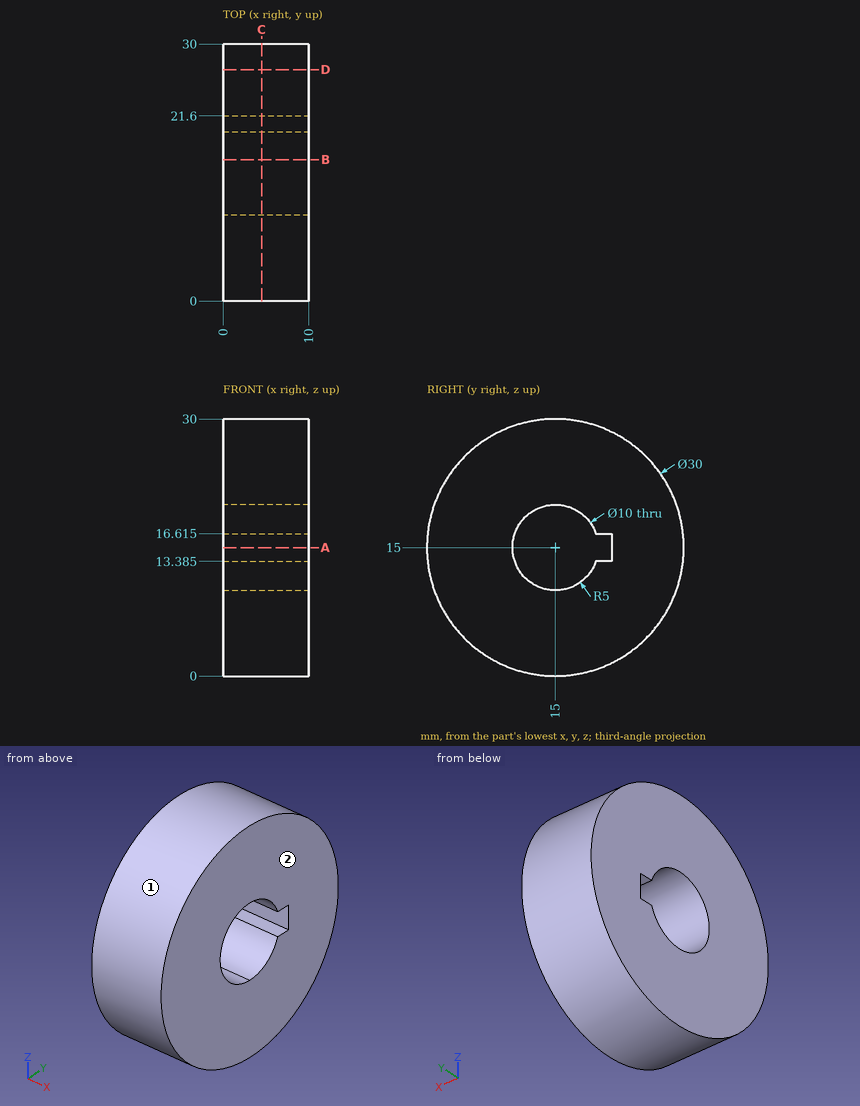
Geometry: see drawing. Coordinates: mm, zero at the bounding-box minimum. Round coordinates to 2 decimals unless told otherwise and drop trailing zeros. Loops run counter-clockwise (first coordinate to the right, second up) from the corner with the lowest first, then second, coordinate; pieces in that order, holes last. Notation, with made-up numbers: (52.5, -30.75) -> (111.5, -30.75) arc R38 cw to (111.5, 7.25) -> close; hole circle Ø5 at (19, 51). An arc over 180 degrees is marked (long way). Use one line per item in the form item = value. Start each with the question number.
Item 1: Mould query, pull axis Y, two halves, no side actions, for the marked faces 1 and 2. Classes: pulls with the +Y half, pulls with the -Y half, needs draft (parallel to the pull), parting line crosses it, or undercut.
Item 2: Section query C-C on x = 4.5. Return the cut outline in (y, z) (3 decimals), then the cut area to 3 significant figures.
Item 3: Section query D-D on y = 27. Return the cut outline in (x, z).
Item 4: Section query B-B on y = 16.5. Return the cut outline in (x, z).
Item 5: Material intervals for L1, parallel to Y at x = 2.5, z = 15; L2, parallel to Y at x = 5, z = 14.25; L3, parallel to Z at x = 9.75, y = 10.5, sorted ascending. Write a range as from..to.
Item 6: Section query A-A on z = 15. Return the cut outline in (x, y).
Item 7: Contact query for flat-ended pins moving along their axis: pin 1 Ø5 at (x, y) = (3.5, 5) entering from +Z; pin 2 Ø4 at (x, z) = (3.5, 19.5) entering from -Y; pin 3 Ø0.6 at (x, y) = (7, 20.5) entering from -Z. Output: stop coordinate, or through.
Ans:
q1.face_1 = parting line crosses it
q1.face_2 = needs draft
q2.outline = circle Ø30 at (15, 15); hole (19.732, 13.385) -> (21.6, 13.385) -> (21.6, 16.615) -> (19.732, 16.615) arc R5 ccw (long way) to start
q2.area = 623 mm^2
q3.outline = (0, 6) -> (10, 6) -> (10, 24) -> (0, 24) -> close
q4.outline = (0, 0.08) -> (10, 0.08) -> (10, 10.23) -> (0, 10.23) -> close; (0, 19.77) -> (10, 19.77) -> (10, 29.92) -> (0, 29.92) -> close
q5.L1 = 0..10, 21.6..30
q5.L2 = 0.02..10.06, 21.6..29.98
q5.L3 = 0.69..12.82, 17.18..29.31
q6.outline = (0, 0) -> (10, 0) -> (10, 10) -> (0, 10) -> close; (0, 21.6) -> (10, 21.6) -> (10, 30) -> (0, 30) -> close
q7.pin_1 = 27.99
q7.pin_2 = 0.21
q7.pin_3 = 0.93
